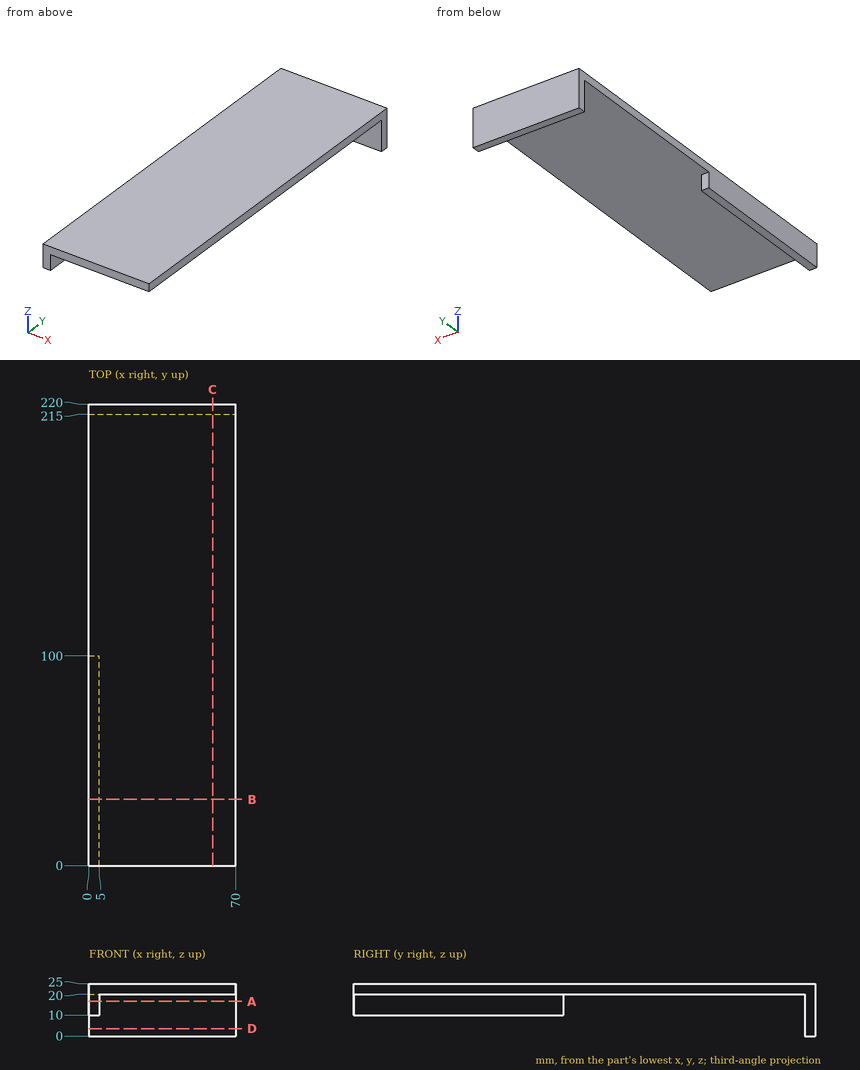
Input: dimensioned drawing with shaded views. Units: mm. Origin: part minimum x, y, z. Coordinates: 2 decimals unless noted, no trailing zeros. Write each loop counter-clockwise with the first axis right and the second up, starting at its lowest first coordinate (ties: lowest second). Pieces come first, ordered by that corner, then holes. Notation, with made-up numbers: (36.5, -2) -> (85.5, -2) arc R19 ccw to (85.5, 17) -> close; hole circle Ø6 at (-38.5, -31.75). An arc over 180 degrees is marked (long way). Return JSON: item names as keys, results as strings. Group by question number.
1) Ray query, line 1 along Z through (x, y) = (20, 136); line 2 along Y through (x, z) = (3, 18); line 3 along Y through (x, z) = (45, 10.25). Return the intervals inside material, ascending.
2) Section query A-A, the plane z = 16.5. Return loops of the section in (x, y).
3) Contact query for flat-ended pins moving along their axis: P1, Ø2, axis at x = 34, z = 7.5, coming from the -Y side; P2, Ø12, axis at x = 46.5, y = 89.5, coming from the -Z side; P3, Ø4, axis at x = 2, y = 60.5, coming from the -Z side. Output: stop coordinate, or through.
4) Section query D-D, the plane z = 3.5. Return loops of the section in (x, y).
5) Section query B-B, the plane y = 31.5. Return loops of the section in (x, z).
6) Section query C-C, the plane x = 59. Return loops of the section in (y, z), plus the area to 3 significant figures.
From the geometry:
{
 "1": {"line 1": "20 to 25", "line 2": "0 to 100, 215 to 220", "line 3": "215 to 220"},
 "2": {"outline": "(0, 0) -> (5, 0) -> (5, 100) -> (0, 100) -> close; (0, 215) -> (70, 215) -> (70, 220) -> (0, 220) -> close"},
 "3": {"P1": "y = 215", "P2": "z = 20", "P3": "z = 10"},
 "4": {"outline": "(0, 215) -> (70, 215) -> (70, 220) -> (0, 220) -> close"},
 "5": {"outline": "(0, 10) -> (5, 10) -> (5, 20) -> (70, 20) -> (70, 25) -> (0, 25) -> close"},
 "6": {"outline": "(0, 20) -> (215, 20) -> (215, 0) -> (220, 0) -> (220, 25) -> (0, 25) -> close", "area": "1,200 mm²"}
}
